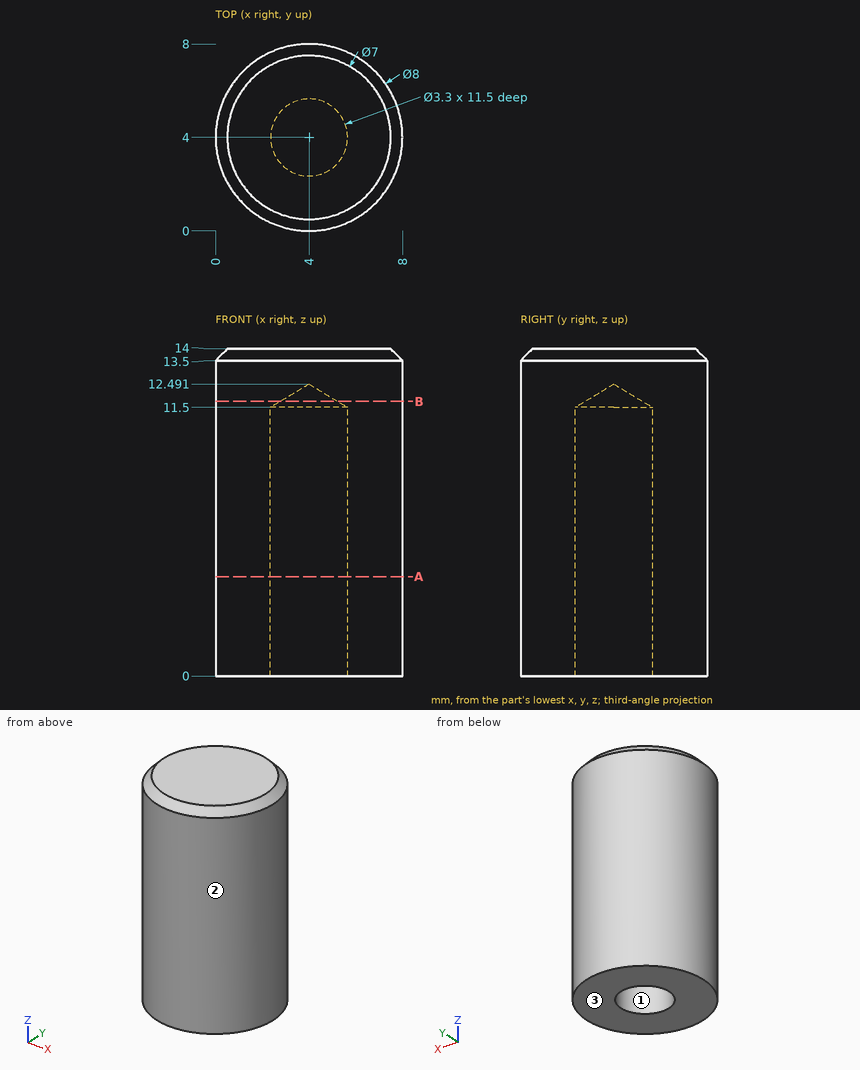
For this review, use the dimensioned drawing (mm, ordinates from the lowest corner) and the shaded views. Coordinates: 2 decimals unless noted, no trailing zeros. Order: outer loops, then holes, each group sorted by start corner. A loop starts at its lowest first (then second) coordinate and runs counter-clockwise, first axis right, second up. Notation, with made-up numbers: (5.5, 15) - (18.5, 15) arc R25 ccw to (18.5, 32) - close; hole circle Ø8 at (-16.5, 82.5). An arc over 180 degrees is marked (long way). Answer as a JSON object with one key per item and string values. Group by question number.
1. We need section B-B on z = 11.75. State the section outline as (x, y) points, then the cut area to 3 significant figures.
2. For probe 1 along Y at (x, z) = (4, 8); probe 2 along X at (y, z) = (4.5, 6.25); probe 3 along X at (y, z) = (5.5, 11) (1 decimal), list the stretches that pass through material, from the lowest coordinate up.
3. We need section A-A on z = 4.25. State the section outline as (x, y) points.
4. Clearance check with flat-ended pins moving along their axes: P1, Ø1, axis at y = 2.5, z = 6.5, coming from the +X side; P2, Ø3, axis at x = 1, z = 8, coming from the +Y side; P3, Ø1, axis at x = 6.5, z = 9.5, coming from the -Y side (1 decimal). State where each tip first meets the part, or that it passes through.
5. The part is to be moulded in two halves that separate along Y. For the marked faces 1, 2 and 3, say which applies: pulls with the +Y half, pulls with the -Y half, needs draft (parallel to the pull), parting line crosses it, or undercut.
Final values:
{
 "1": {"outline": "circle Ø8 at (4, 4); hole circle Ø2.47 at (4, 4)", "area": "45.5 mm²"},
 "2": {"probe 1": "0 to 2.35, 5.65 to 8", "probe 2": "0.03 to 2.43, 5.57 to 7.97", "probe 3": "0.3 to 3.3, 4.7 to 7.7"},
 "3": {"outline": "circle Ø8 at (4, 4); hole circle Ø3.3 at (4, 4)"},
 "4": {"P1": "x = 7.87", "P2": "y = 7.71", "P3": "y = 0.5"},
 "5": {"face 1": "undercut", "face 2": "parting line crosses it", "face 3": "needs draft"}
}
